Autodesk Inventor part; units mm, degrees
ref_plane "YZ Plane" through (0, 0, 0) normal (1, 0, 0) x (0, 1, 0)
ref_plane "XZ Plane" through (0, 0, 0) normal (0, 1, 0) x (-1, 0, 0)
ref_plane "XY Plane" through (0, 0, 0) normal (0, 0, 1) x (1, 0, 0)
sketch "Sketch1" plane through (0, 0, 0) normal (0, 1, 0) x (-1, 0, 0)
  line L0 (1.9169, 3.0365) -> (-11.4831, 3.0365)
  line L1 (-11.4831, 3.0365) -> (-11.4831, -12.9635)
  line L2 (-11.4831, -12.9635) -> (1.9169, -12.9635)
  line L3 (1.9169, -12.9635) -> (1.9169, 3.0365)
  point P0 (0, 0)
  dimension "d0" = 13.4
  dimension "d1" = 16
extrude "Extrusion1" add sketch "Sketch1" along normal blind 21.4
sketch "Sketch2" plane through (0, 21.4, 0) normal (0, 1, 0) x (1, 0, 0)
  line L0 (0.9831, -1.0365) -> (0.9831, 10.9635)
  line L1 (11.4831, 12.9635) -> (-1.9169, 12.9635)
  line L2 (0.9831, 10.9635) -> (7.9831, 10.9635)
  line L3 (7.9831, 10.9635) -> (7.9831, 8.4635)
  line L4 (7.9831, 8.4635) -> (10.9831, 8.4635)
  line L5 (10.9831, 8.4635) -> (10.9831, 1.4635)
  line L6 (10.9831, 1.4635) -> (7.9831, 1.4635)
  line L7 (7.9831, 1.4635) -> (7.9831, -1.0365)
  line L8 (7.9831, -1.0365) -> (0.9831, -1.0365)
  line L9 (-1.9169, -3.0365) -> (11.4831, -3.0365)
  line L10 (-1.9169, 12.9635) -> (-1.9169, -3.0365)
  point P0 (0, 0)
  dimension "d4" = 12
  dimension "d5" = 7
  dimension "d6" = 7
  dimension "d7" = 3
  dimension "d8" = 7
  dimension "d9" = 2.5
  dimension "d10" = 2.5
  dimension "d11" = 2
  dimension "d12" = 2
  dimension "d13" = 2.9
extrude "Extrusion2" cut sketch "Sketch2" against normal blind 12
sketch "Sketch3" plane through (11.4831, 0, 3.0365) normal (1, 0, 0) x (0, 0, -1)
  circle A0 centre (13.7, 12.4) radius 1.5
  circle A1 centre (2.3, 12.4) radius 1.5
  line L0 (0, 21.4) -> (16, 21.4)
  line L1 (0, 0) -> (0, 21.4)
  line L2 (16, 0) -> (16, 21.4)
  point P0 (3.0365, 0)
  dimension "d16" = 3
  dimension "d17" = 3
  dimension "d18" = 9
  dimension "d19" = 9
  dimension "d20" = 2.3
  dimension "d21" = 2.3
extrude "Extrusion3" add sketch "Sketch3" along normal blind 4
sketch "Sketch4" plane through (11.4831, 0, 3.0365) normal (1, 0, 0) x (0, 0, -1)
  circle A0 centre (3.6, 4.2) radius 0.2
  circle A1 centre (6, 4.2) radius 0.2
  line L0 (0, 0) -> (0, 21.4)
  circle A2 centre (8.4, 4.2) radius 0.2
  circle A3 centre (10.8, 4.2) radius 0.2
  line L1 (0, 0) -> (16, 0)
  line L2 (0.3816, 1.4) -> (15.1957, 1.4)
  circle A4 centre (5, 1.4) radius 0.2
  circle A5 centre (7.4, 1.4) radius 0.2
  circle A6 centre (9.8, 1.4) radius 0.2
  circle A7 centre (12.2, 1.4) radius 0.2
  point P0 (3.0365, 0)
  dimension "d24" = 0.4
  dimension "d25" = 0.4
  dimension "d26" = 3.6
  dimension "d27" = 2.4
  dimension "d28" = 0.4
  dimension "d29" = 0.4
  dimension "d30" = 2.4
  dimension "d31" = 2.4
  dimension "d32" = 0
  dimension "d33" = 0
  dimension "d34" = 0
  dimension "d35" = 4.2
  dimension "d36" = 1.4
  dimension "d37" = 0.4
  dimension "d38" = 0.4
  dimension "d39" = 0.4
  dimension "d40" = 0.4
  dimension "d41" = 1.4
  dimension "d42" = 2.4
  dimension "d43" = 2.4
  dimension "d44" = 2.4
extrude "Extrusion4" add sketch "Sketch4" along normal blind 3.4
equation "\"d21\" = d20"
properties part number "rj45"
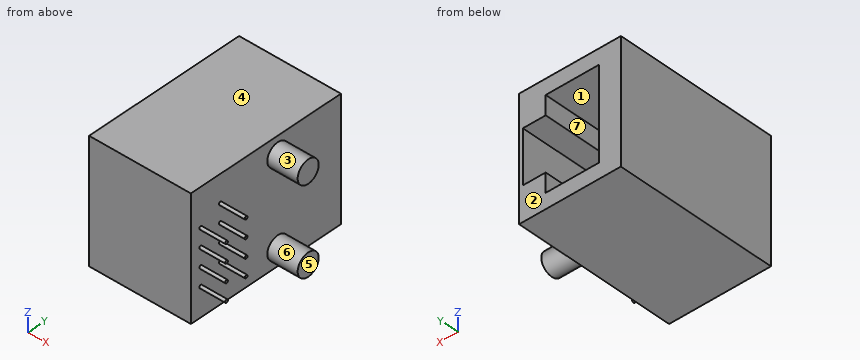
Verification items for the finished model (mm, model axes). Face numbers are marked on the shaded views. A direction names the side the tool comes from. Coordinates: 2 decimals unless noted, no trailing zeros. Write each loop counter-clockwise with the first axis right and the second up, starting at its lowest first coordinate (ties: lowest second). Pieces come first, ordered by that corner, then holes. Notation, with made-up numbers: M 52,18 L 65,18 A23 ccw 65,42 Z; hole C -21.5,54 d4. An arc over 180 degrees is marked long. Use a Markdown table: item, result.
Q1. Sectioned sample at A-A, the plane x = 14. Count the separate pieces of the cut face and the enclosed holes in it, plus the area to 3 significant figures.
Reply:
| item | result |
|---|---|
| separate pieces | 10 |
| enclosed holes | 0 |
| area | 15.1 mm² |
Q2. Thickness scan on line 1 (Z direction, x = 2.25, y = 20.25); line 2 (Z direction, x = 10, y = 11.5); line 3 (X direction, y = 9.5, z = 1). Record the ranges inside material, lowest first.
Reply:
| item | result |
|---|---|
| line 1 | z = -12.96 to -10.96, 1.04 to 3.04 |
| line 2 | z = -12.96 to -8.46, -1.46 to 3.04 |
| line 3 | x = -1.92 to 0.98, 7.98 to 11.48 |
Q3. Sectioned sample at D-D, the plane x = 4.5. Record the boundary of the cut face in (y, z).
Reply:
| item | result |
|---|---|
| outline | M 0,-12.96 L 21.4,-12.96 L 21.4,-10.96 L 9.4,-10.96 L 9.4,1.04 L 21.4,1.04 L 21.4,3.04 L 0,3.04 Z |
Q4. Draft check along Z on the marked faces 1, 2, 3 and 4. Enter one of: +Z half, -Z half, draft (parallel to the pull), parting line (faces both ways), or undercut.
Reply:
| item | result |
|---|---|
| face 1 | undercut |
| face 2 | draft |
| face 3 | undercut |
| face 4 | +Z half |
Q5. Set-up check for the marked faces 5, 6 and 7: record each of +Z, -Z, +X, -X, +Y, -Y from which the full face is reachable in a straight line by a thin tool's end or side.
Reply:
| item | result |
|---|---|
| face 5 | +Z, -Z, +X, +Y, -Y |
| face 6 | +X |
| face 7 | +Y |
Q6. Go/stop test with flat-tipped pins: P1, Ø3.5, axis at y = 16.5, z = -6, coming from the +X side; P2, Ø4, axis at x = 4, z = -2, coming from the +Y side; P3, Ø1, axis at x = 10.5, z = -11, coming from the -Y side; P4, Ø1, axis at x = 13.5, y = 13.5, coming from the -Z side. Record where each tip stops, or that it passes through.
Reply:
| item | result |
|---|---|
| P1 | stops at x = 11.48 |
| P2 | stops at y = 9.4 |
| P3 | stops at y = 0 |
| P4 | stops at z = -12.04 |
Q7. Sectioned sample at B-B, the plane y = 10.5. Record the boundary of the cut face in (x, z).
Reply:
| item | result |
|---|---|
| outline | M -1.92,-12.96 L 11.48,-12.96 L 11.48,3.04 L -1.92,3.04 Z; hole M 0.98,-10.96 L 7.98,-10.96 L 7.98,-8.46 L 10.98,-8.46 L 10.98,-1.46 L 7.98,-1.46 L 7.98,1.04 L 0.98,1.04 Z |
Q8. Sectioned sample at C-C, the plane z = -6. Record the boundary of the cut face in (x, y), plus the area to 3 significant figures.
Reply:
| item | result |
|---|---|
| outline | M -1.92,0 L 11.48,0 L 11.48,21.4 L 10.98,21.4 L 10.98,9.4 L 0.98,9.4 L 0.98,21.4 L -1.92,21.4 Z |
| area | 167 mm² |
